Geometry: see drawing. Coordinates: mm, zero at the bounding-box minimum. A direction names the side the tool comes from. Round coordinates to 2 decimals unless told otherwise and drop trailing zeros. Loops run counter-clockwise (first coordinate to the right, second up) from the corner with the lowest first, then second, coordinate; pieces in that order, holes last.
(1) Set-up query: the marked faces 1, 2 and 3. Return all of +Z, -Z, +X, -X, +Y, -Y with unobstructed straight access to the full face (end or side cutting, diameter ignored); none if empty.
(2) Section C-C, the plane x = 18.5. Return the cut outline in (y, z), plus the area to 3 significant figures.
(3) First-contact query: pin 1 Ø7.5 at (x, y) = (32, 51) entering from -Z; pin 2 Ø9 at (x, y) = (23.5, 56) entering from +Z; pin 3 Ø3 at (x, z) = (25, 29) entering from -Y. Flat tips, straight axial feed; report the tip coordinate or a pass-through.
(4) Section A-A, the plane y = 38. Return the cut outline in (x, z), plus the area to 3 significant figures.
(5) Material intervals for probe 1 along X at (y, z) = (43.5, 45); probe 2 along Y at (x, z) = (42, 13.5); probe 3 along Z at (x, y) = (3, 20) (1 decimal), sorted ascending.
(6) Mould query, pull axis X, two halves, no side actions, for the marked faces 4, 5 and 6. Classes: pulls with the +X half, pulls with the -X half, needs draft (parallel to the pull), parting line crosses it, or undercut.
(7) Section D-D, the plane y = 20.32. Return the cut outline in (x, z), plus the area to 3 significant figures.
(8) Section B-B, the plane z = 42. Return the cut outline in (x, y) (1 decimal), plus the area to 3 significant figures.
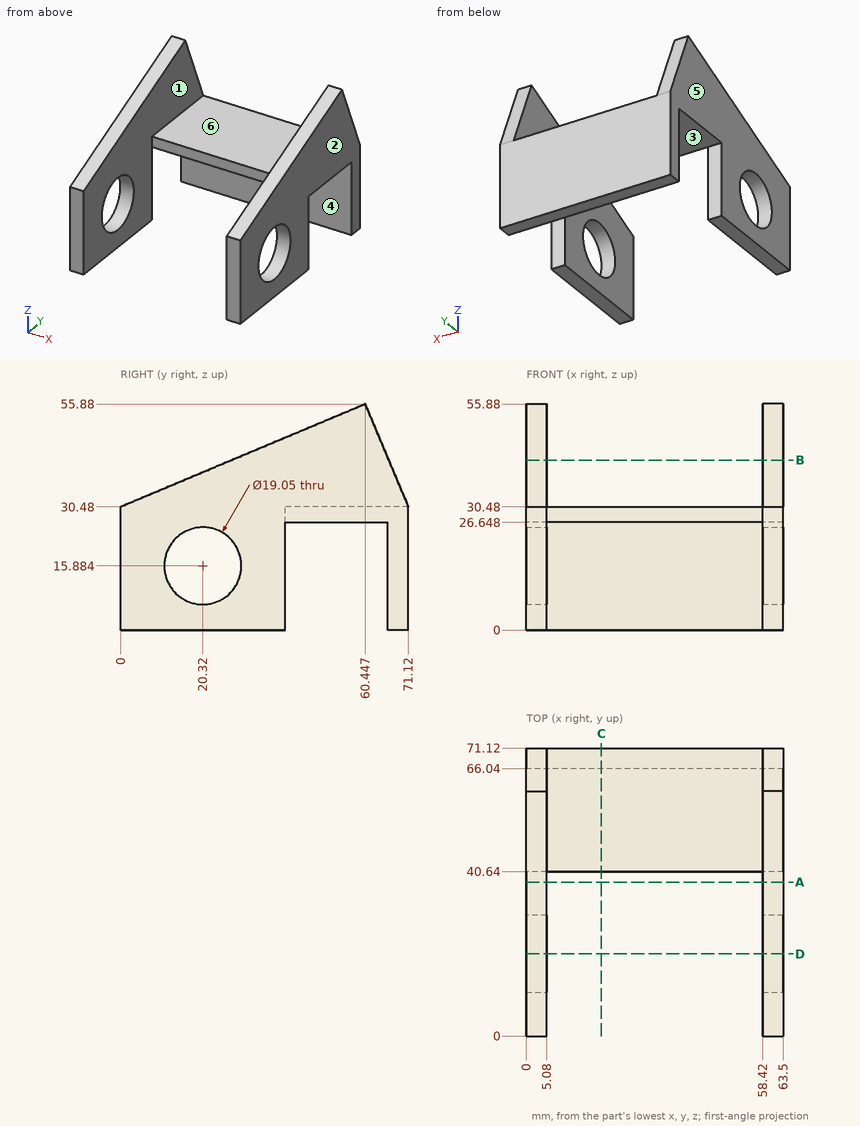
Output values:
1. face 1: +Z, -Y
1. face 2: +Z, -Z, +X, +Y, -Y
1. face 3: -Z, +X, -X
2. outline: (40.64, 26.65) - (66.04, 26.65) - (66.04, 0) - (71.12, 0) - (71.12, 30.48) - (40.64, 30.48) - close
2. area: 252 mm2
3. pin 1: stops at z = 26.65
3. pin 2: stops at z = 30.48
3. pin 3: stops at y = 40.64
4. outline: (0, 0) - (5.08, 0) - (5.08, 46.45) - (0, 46.45) - close; (58.42, 0) - (63.5, 0) - (63.5, 46.45) - (58.42, 46.45) - close
4. area: 472 mm2
5. probe 1: x = 0 to 5.08, 58.42 to 63.5
5. probe 2: y = 66.04 to 71.12
5. probe 3: z = 0 to 6.4, 25.4 to 38.9
6. face 4: needs draft
6. face 5: pulls with the -X half
6. face 6: undercut
7. outline: (0, 0) - (5.08, 0) - (5.08, 6.36) - (0, 6.36) - close; (0, 25.41) - (5.08, 25.41) - (5.08, 39.02) - (0, 39.02) - close; (58.42, 0) - (63.5, 0) - (63.5, 6.36) - (58.42, 6.36) - close; (58.42, 25.41) - (63.5, 25.41) - (63.5, 39.02) - (58.42, 39.02) - close
7. area: 203 mm2
8. outline: (0, 27.4) - (5.1, 27.4) - (5.1, 66.3) - (0, 66.3) - close; (58.4, 27.4) - (63.5, 27.4) - (63.5, 66.3) - (58.4, 66.3) - close
8. area: 395 mm2
